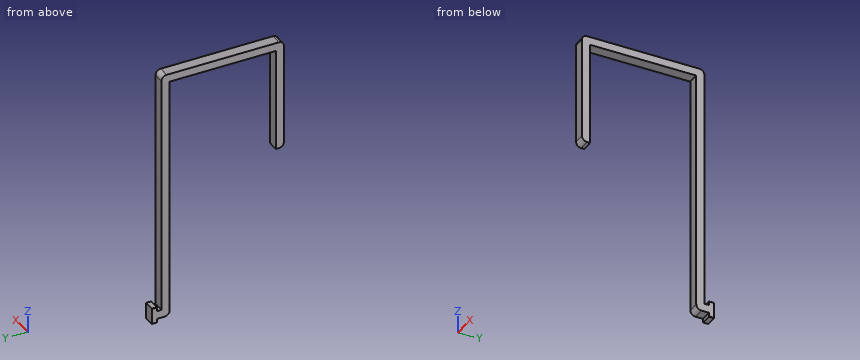
```python
from build123d import *

# Parameters (mm, degrees)
F1_DEPTH = 5.5
F2_R     = 0.254
F3_R     = 2.54


with BuildPart() as f1:
    # F0 (on Right) → F1 (new body)
    with BuildSketch(Plane.YZ):
        Polygon((0, 0), (0, -29.4), (0, -54.8), (4, -54.8), (4, -4), (56.07, -4), (56.07, -125), (60.07, -125), (62.32, -125), (62.32, -127), (64.77, -127), (64.77, -119), (62.32, -119), (62.32, -121), (60.07, -121), (60.07, 0), align=None)
    extrude(amount=F1_DEPTH)

    # F2
    f2_edges = [f1.edges().sort_by_distance(p)[0] for p in [
        (5.5, 63.545, -119),
        (5.5, 63.545, -127),
        (0, 63.545, -119),
        (0, 63.545, -127),
    ]]
    fillet(f2_edges, radius=F2_R)

    # F3
    f3_edges = [f1.edges().sort_by_distance(p)[0] for p in [
        (2.75, 60.07, 0),
        (2.75, 0, 0),
        (2.75, 56.07, -125),
        (2.75, 0, -54.8),
    ]]
    fillet(f3_edges, radius=F3_R)


solid = f1.part
```
Work out the finished part from the listing and answer in its coordinate system (mm). Coordinates: 2 decimals unless noted, no trailing zeros. Order: outer loops, then holes, each group sorted by start corner. A loop starts at its lowest first (then second) coordinate and runs counter-clockwise, first axis right, second up. Notation, with made-up numbers: M -31,12.25 L -21,12.25 A29 cw -21,42.25 Z; hole C 38,-7.75 d8. An arc over 180 degrees is marked long. Use CSV: the item, a comma, the result in double quotes.
1) Section A-A on z = -20.5 is taken. Write down the section's boundary in (x, y).
Worked out:
outline,"M 0,0 L 5.5,0 L 5.5,4 L 0,4 Z; M 0,56.07 L 5.5,56.07 L 5.5,60.07 L 0,60.07 Z"
2) Consider line 1 (Y direction, x = 2.9, z = -39.5); line 2 (Y direction, x = 4.25, z = -85); line 3 (Z direction, x = 5.1, y = 29). Determine where each line is inside the solid, lowest interval first. Write a range as [from, to].
Worked out:
line 1,"y = [0, 4], [56.07, 60.07]"
line 2,"y = [56.07, 60.07]"
line 3,"z = [-4, 0]"
3) Section D-D on z = -59 is taken. Write down the section's boundary in (x, y).
Worked out:
outline,"M 0,56.07 L 5.5,56.07 L 5.5,60.07 L 0,60.07 Z"
4) Section B-B on x = 1.75 is taken. Write down the section's boundary in (y, z).
Worked out:
outline,"M 0,-52.26 A2.54 ccw 2.54,-54.8 L 4,-54.8 L 4,-4 L 56.07,-4 L 56.07,-122.46 A2.54 ccw 58.61,-125 L 62.32,-125 L 62.32,-127 L 64.77,-127 L 64.77,-119 L 62.32,-119 L 62.32,-121 L 60.07,-121 L 60.07,-2.54 A2.54 ccw 57.53,0 L 2.54,0 A2.54 ccw 0,-2.54 Z"
5) Section C-C on y = 45.5 is taken. Write down the section's boundary in (x, z).
Worked out:
outline,"M 0,-4 L 5.5,-4 L 5.5,0 L 0,0 Z"
6) Flat-ended cylindrical pins translate along their axes: pin 1 Ø3 at (x, y) = (0.5, 42.5) entering from -Z; pin 2 Ø1.6 at (x, y) = (4, 3) entering from -Z; pin 3 Ø1 at (x, z) = (3.5, -120) entering from -Y. Find the tip coordinate at first contact, or state that the pin passes through.
Worked out:
pin 1,"stops at z = -4"
pin 2,"stops at z = -54.8"
pin 3,"stops at y = 56.07"
